from build123d import *

# Parameters (mm, degrees)
BOSS_EXTRUDE1_DEPTH = 152.4
SKETCH2_R           = 2.54
CUT_EXTRUDE2_DEPTH  = 31.75


with BuildPart() as part:
    # Sketch1 → Boss-Extrude1 (new body)
    with BuildSketch(Plane(origin=(0, 0, 0), x_dir=(1, 0, 0), z_dir=(0, 1, 0))):
        Polygon((0, 0), (31.75, 0), (31.75, 31.75), (28.575, 31.75), (28.575, 3.175), (3.175, 3.175), (3.175, 31.75), (0, 31.75), align=None)
    extrude(amount=BOSS_EXTRUDE1_DEPTH)

    # Sketch2 → Cut-Extrude2 (cut)
    with BuildSketch(Plane(origin=(31.75, 0, 0), x_dir=(0, 0, -1), z_dir=(1, 0, 0))):
        with Locations((24.60625, 6.35)):
            Circle(SKETCH2_R)
        with Locations((10.31875, 6.35)):
            Circle(SKETCH2_R)
        with Locations((24.60625, 146.05)):
            Circle(SKETCH2_R)
        with Locations((10.31875, 146.05)):
            Circle(SKETCH2_R)
    extrude(amount=-CUT_EXTRUDE2_DEPTH, mode=Mode.SUBTRACT)


solid = part.part
Check sheet for the modelled part. Datum: model origin and axes. Units: mm. A direction names the side the tool comes from. Coordinates: 2 decimals unless noted, no trailing zeros. Write each loop counter-clockwise with the first axis right and the second up, starting at its lowest first coordinate (ties: lowest second). Pieces come first, ordered by that corner, then holes.
Item 1: Cross-section at A-A on y = 146.05. Record the boundary of the cut face in (x, z) (3 decimals).
Numbers:
outline: (0, -31.75) - (3.175, -31.75) - (3.175, -27.146) - (0, -27.146) - close; (0, -22.066) - (3.175, -22.066) - (3.175, -12.859) - (0, -12.859) - close; (0, -7.779) - (3.175, -7.779) - (3.175, -3.175) - (28.575, -3.175) - (28.575, -7.779) - (31.75, -7.779) - (31.75, 0) - (0, 0) - close; (28.575, -31.75) - (31.75, -31.75) - (31.75, -27.146) - (28.575, -27.146) - close; (28.575, -22.066) - (31.75, -22.066) - (31.75, -12.859) - (28.575, -12.859) - close
Item 2: Depth check by flat-ended pin: pin 1 Ø4.5 at (y, z) = (6.35, -10.32) entering from -X; pin 2 Ø3 at (x, y) = (5.5, 63) entering from -Z (3 decimals); pin 3 Ø2 at (x, y) = (15.5, 84) entering from +Z. Enter the tip coordinate at first touch or a pass-through.
Numbers:
pin 1: passes through
pin 2: stops at z = -3.175
pin 3: stops at z = 0
Item 3: Scan lines: probe 1 along Z at (x, y) = (30, 146); probe 2 along X at (y, z) = (71.5, -5) (3 decimals); probe 3 along Z at (x, y) = (14, 99.5) (3 decimals). Record each from-to range of solid material in increasing order.
Numbers:
probe 1: z = -31.75 to -27.15, -22.07 to -12.86, -7.78 to 0
probe 2: x = 0 to 3.175, 28.575 to 31.75
probe 3: z = -3.175 to 0
Item 4: Cross-section at C-C on x = 17. Record the boundary of the cut face in (y, z) (3 decimals).
Numbers:
outline: (0, -3.175) - (152.4, -3.175) - (152.4, 0) - (0, 0) - close
Item 5: Access from +Z, -Z, +X, -X, +Y, -Y to the whole of each face (thin tool, end or side, straight path). Record for faces 1 (the face through (28.575, 75, -18)), 2 (the face through (31.75, 75, -16)).
Numbers:
face 1: -Z, +Y, -Y
face 2: +Z, -Z, +X, +Y, -Y
Item 6: Cross-section at B-B on y = 122.5. Record the boundary of the cut face in (x, z) (3 decimals), then the cut area to 3 significant figures.
Numbers:
outline: (0, -31.75) - (3.175, -31.75) - (3.175, -3.175) - (28.575, -3.175) - (28.575, -31.75) - (31.75, -31.75) - (31.75, 0) - (0, 0) - close
area: 282 mm2
Item 7: Mould release check, pull along X, two halves, no side actions. Record for faces 3 (the face through (16, 75, -3.175)), 4 (the face through (16, 0, -3)), 5 (the face through (0, 75, -16)): released by +X, released by -X, zero draft, split by the parting line, or undercut.
Numbers:
face 3: undercut
face 4: zero draft
face 5: released by -X
